Autodesk Inventor part; units mm, degrees
ref_plane "YZ Plane" through (0, 0, 0) normal (1, 0, 0) x (0, 1, 0)
ref_plane "XZ Plane" through (0, 0, 0) normal (0, 1, 0) x (-1, 0, 0)
ref_plane "XY Plane" through (0, 0, 0) normal (0, 0, 1) x (1, 0, 0)
sketch "スケッチ1" plane through (0, 0, 0) normal (1, 0, 0) x (0, 1, 0)
  circle A0 centre (0, 0) radius 10
  circle A1 centre (0, -10) radius 1.35
  circle A2 centre (8.6603, 5) radius 1.35
  circle A3 centre (-8.6603, 5) radius 1.35
  circle A4 centre (0, 0) radius 5
  line L0 (0, 0) -> (0, 50)
  circle A5 centre (0, 50) radius 22.5
  circle A6 centre (0, 0) radius 14
  line L1 (-14, 0) -> (-22.5, 50)
  line L2 (14, 0) -> (22.5, 50)
  line L3 (0, -14) -> (-11.62, -14)
  line L4 (-11.62, -14) -> (-14, 0)
  line L5 (0, -14) -> (11.62, -14)
  line L6 (11.62, -14) -> (14, 0)
  line L7 (0, 20) -> (-17.4, 20)
  line L8 (0, 20) -> (17.4, 20)
  dimension "d0" = 20
  dimension "d1" = 2.7
  dimension "d4" = 360
  dimension "d6" = 10
  dimension "d7" = 50
  dimension "d8" = 45
  dimension "d9" = 28
extrude "押し出し1" add sketch "スケッチ1" along normal blind 4 contours A0 A1 A3 A2 | A6 L6 L4 | A6 L1 L7 L0 | L0 L8 L2 A6 | L6 L5 A6 | A6 L3 L4
sketch "スケッチ2" plane through (0, -17.4, 20) normal (0, 0, 1) x (1, 0, 0)
  line L0 (0, 17.4) -> (30, 17.4)
  circle A0 centre (30, 17.4) radius 22.5
  circle A1 centre (30, 17.4) radius 18.5
  circle A2 centre (30, 17.4) radius 14.25
  circle A3 centre (48.5, 17.4) radius 1.35
  circle A4 centre (20.75, 33.4215) radius 1.35
  circle A5 centre (20.75, 1.3785) radius 1.35
  line L1 (0, 29.02) -> (0, 34.8)
  line L2 (0, 0) -> (0, 5.78)
  line L3 (0, 34.8) -> (0, 0)
  line L4 (4, 29.02) -> (4, 34.8)
  line L5 (4, 34.8) -> (7, 34.8)
  line L6 (7, 34.8) -> (30, 39.9)
  line L7 (4, 0) -> (4, 5.78)
  line L8 (4, 0) -> (7, 0)
  line L9 (7, 0) -> (30, -5.1)
  line L10 (4, 0) -> (0, 0)
  line L11 (0, 34.8) -> (4, 34.8)
  line L12 (0, 0) -> (0, 34.8)
  line L13 (0, 34.8) -> (4, 34.8)
  dimension "d14" = 37
  dimension "d12" = 30
  dimension "d13" = 45
  dimension "d15" = 28.5
  dimension "d16" = 2.7
  dimension "d19" = 360
  dimension "d21" = 3
  dimension "d22" = 3
extrude "押し出し2" add sketch "スケッチ2" along normal blind 4 contours L3 L1 L11 L5 L6 A0 L0 | L0 A0 L9 L8 L10 L2 L3 | A1 A4 A3 A5 | A0 L6 L9
fillet "フィレット1" radius 3 2 edges at (4, 0, 20) (0, 0, 24)
fillet "フィレット2" radius 3 2 edges at (2, -11.62, -14) (2, 11.62, -14)
sketch "スケッチ7" plane through (0, -17.4, 24) normal (0, 0, 1) x (1, 0, 0)
  circle A0 centre (30, 17.4) radius 14.25
  line L0 (30, 17.4) -> (182.95, 17.4)
  line L1 (30, 17.4) -> (182.95, 17.4) construction
  circle A1 centre (182.95, 17.4) radius 3.5
  circle A2 centre (182.95, 17.4) radius 10
  line L2 (182.95, 27.4) -> (50.1556, 27.4)
  arc A3 (30, -5.1) -> (30, 39.9) centre (30, 17.4) ccw
  line L3 (182.95, 27.4) -> (315.7444, 27.4) construction
  line L4 (182.95, 7.4) -> (50.1556, 7.4)
  point P0 (0, 17.4)
  dimension "d55" = 152.95
  dimension "d56" = 0
  dimension "d57" = 7
  dimension "d58" = 20
  dimension "d59" = 180
extrude "押し出し7" add sketch "スケッチ7" against normal blind 4 contours A3 L2 A2 L0 | L0 A2 L4 A3 | A2
sketch "スケッチ8" plane through (0, -17.4, 24) normal (0, 0, 1) x (1, 0, 0)
  circle A0 centre (20.75, 33.4215) radius 1.35
  circle A1 centre (20.75, 33.4215) radius 2.5
  circle A2 centre (48.5, 17.4) radius 1.35
  circle A3 centre (48.5, 17.4) radius 2.5
  circle A4 centre (20.75, 1.3785) radius 1.35
  circle A5 centre (20.75, 1.3785) radius 2.5
  point P0 (0, 17.4)
  dimension "d63" = 5
  dimension "d64" = 5
  dimension "d65" = 5
extrude "押し出し8" cut sketch "スケッチ8" against normal blind 2 contours A0 | A1 | A3 | A4 | A5
fillet "フィレット4" radius 2 1 edges at (50.1556, 10, 22)
sketch "スケッチ11" plane through (0, -17.4, 24) normal (0, 0, 1) x (1, 0, 0)
  line L0 (51.36, 27.4) -> (182.95, 27.4)
  line L1 (182.95, 27.4) -> (202.95, 27.4)
  arc A0 (182.95, 7.4) -> (182.95, 27.4) centre (182.95, 17.4) ccw
  line L2 (182.95, 7.4) -> (207.95, 7.4)
  line L3 (207.95, 13.4) -> (207.95, 22.4)
  line L4 (207.95, 7.4) -> (221.95, 7.4)
  line L5 (222.95, 8.4) -> (222.95, 26.4)
  line L6 (221.95, 27.4) -> (218.95, 27.4)
  line L7 (217.95, 26.4) -> (217.95, 13.4)
  line L8 (216.95, 12.4) -> (208.95, 12.4)
  arc A1 (222.95, 26.4) -> (221.95, 27.4) centre (221.95, 26.4) ccw
  arc A2 (218.95, 27.4) -> (217.95, 26.4) centre (218.95, 26.4) ccw
  arc A3 (221.95, 7.4) -> (222.95, 8.4) centre (221.95, 8.4) ccw
  arc A4 (216.95, 12.4) -> (217.95, 13.4) centre (216.95, 13.4) ccw
  arc A5 (207.95, 13.4) -> (208.95, 12.4) centre (208.95, 13.4) ccw
  arc A6 (207.95, 22.4) -> (202.95, 27.4) centre (202.95, 22.4) ccw
  point P0 (0, 17.4)
  point P1 (207.95, 27.4)
  point P2 (222.95, 7.4)
  point P3 (222.95, 27.4)
  point P4 (217.95, 27.4)
  point P5 (217.95, 12.4)
  dimension "d83" = 25
  dimension "d84" = 15
  dimension "d85" = 20
  dimension "d86" = 5
  dimension "d87" = 15
  dimension "d88" = 1
  dimension "d89" = 5
extrude "押し出し11" add sketch "スケッチ11" against normal blind 4
properties part number "motor_holder_2" material "ABS プラスチック"
CAD build for the part. Positions are in the model's coordinates, mm. A direction names the side the tool comes from. Round coordinates to 2 decimals unless told otherwise and drop trailing zeros. Loops run counter-clockwise (first coordinate to the right, second up) from the corner with the lowest first, then second, coordinate; pieces in that order, holes last.
(1) Two-plate mould, pull along X, no slides. Class faces 5 (the cylindrical face through (179.453, 0.154, 22.028)), 6 (the cylindrical face through (42.007, -19.029, 21.972)), 7 (the flat face through (217.95, 3, 22)), 8 (the flat face through (126, 10, 22)): +X half, -X half, draft (parallel to the pull), parting line (faces both ways), or undercut.
(2) Cut at C-C (x = 150.5). Give the cut face in (y, z).
(3) Drop flat-ended pins along their axis: pin 1 (4 mm diameter, centred on x = 20.75, y = 16.02, fed in from +Z); pin 2 (6.5 mm diameter, centred on x = 20.75, y = -16.02, fed in from -Z); pin 3 (3 mm diameter, centred on x = 213.5, z = 22, fed in from +Y); pin 4 (2 mm diameter, centred on y = -11, z = -0.5, fed in from -X). Give the stop position or say it passes through.
(4) Which spindle directions (+Z, -Z, +X, -X, +Y, -Y) get a long thin tool onto all of the face, cutting with end or side? Do faces 1 (the flat face through (207.95, 0, 22)), 2 (the flat face through (22, 15, 22)), 3 (the flat face through (4, -0.2, 5.2)), 4 (the flat face through (135, -10, 22)). Say none if no direction does.
(5) Cut at B-B (z = 11). Give the cut face in (x, y).
(6) Cut at A-A (x = 182.95). Give the cut face in (y, z), plus the area to 3 significant figures.
(7) Wall check: line 1 along Z through (x, y) = (1, 0); line 2 along Y through (x, z) = (20.75, 21.3); line 3 along X through (y, z) = (3.5, 14). Give the ranges that are in metal, low to high.
Findings below:
1. face 5: undercut
1. face 6: +X half
1. face 7: undercut
1. face 8: draft
2. outline: (-10, 20) - (10, 20) - (10, 24) - (-10, 24) - close
3. pin 1: stops at z = 22
3. pin 2: stops at z = 20
3. pin 3: stops at y = -5
3. pin 4: stops at x = 0
4. face 1: +Z, -Z, +Y
4. face 2: +Z
4. face 3: -Z, +X, +Y, -Y
4. face 4: +Z, -Z, +X, -Y
5. outline: (0, -15.87) - (4, -15.87) - (4, 15.87) - (0, 15.87) - close
6. outline: (-10, 20) - (-3.5, 20) - (-3.5, 24) - (-10, 24) - close; (3.5, 20) - (10, 20) - (10, 24) - (3.5, 24) - close
6. area: 52.0 mm2
7. line 1: z = -14 to -11.35, -8.65 to -5, 5 to 23.24
7. line 2: y = -20.45 to -17.37, -14.67 to -10.84, 10.84 to 14.67, 17.37 to 20.45
7. line 3: x = 0 to 4
